```python
from build123d import *

# Parameters (mm, degrees)
SKETCH5_R             = 7
BOSS_EXTRUDE2_DEPTH   = 9.8
SKETCH6_R             = 10
BOSS_EXTRUDE3_DEPTH   = 7.2
M8_TAPPED_HOLE2_D     = 6.8
M8_TAPPED_HOLE2_DEPTH = 17
M8_TAPPED_HOLE2_TIP   = 2.042926105
BOSS_EXTRUDE5_DEPTH   = 8
SKETCH12_R            = 2.75
CUT_EXTRUDE6_DEPTH    = 9
M2_TAPPED_HOLE1_D     = 1.6
M2_TAPPED_HOLE1_DEPTH = 5.2
M2_TAPPED_HOLE1_TIP   = 0.480688495


with BuildPart() as part:
    # Sketch5 → Boss-Extrude2 (new body)
    with BuildSketch(Plane(origin=(0, 0, 0), x_dir=(1, 0, 0), z_dir=(0, 1, 0))):
        Circle(SKETCH5_R)
    extrude(amount=BOSS_EXTRUDE2_DEPTH)

    # Sketch6 → Boss-Extrude3 (add)
    with BuildSketch(Plane(origin=(0, 9.8, 0), x_dir=(1, 0, 0), z_dir=(0, 1, 0))):
        Circle(SKETCH6_R)
    extrude(amount=BOSS_EXTRUDE3_DEPTH)

    # M8 Tapped Hole2
    with Locations(Plane(origin=(0, 0, 0), x_dir=(-1, 0, 0), z_dir=(0, -1, 0))):
        with Locations((0, 0)):
            Hole(M8_TAPPED_HOLE2_D / 2, depth=M8_TAPPED_HOLE2_DEPTH)
            with Locations((0, 0, -(M8_TAPPED_HOLE2_DEPTH + M8_TAPPED_HOLE2_TIP / 2))):  # 118° drill point
                Cone(0, M8_TAPPED_HOLE2_D / 2, M8_TAPPED_HOLE2_TIP, mode=Mode.SUBTRACT)

    # Sketch11 → Boss-Extrude5 (add)
    with BuildSketch(Plane(origin=(0, 17, 0), x_dir=(1, 0, 0), z_dir=(0, 1, 0))):
        with BuildLine():
            Line((-5.5, 2.397915762), (-5.5, -2.397915762))
            ThreePointArc((-5.5, -2.397915762), (6, 0), (-5.5, 2.397915762))
        make_face()
    extrude(amount=BOSS_EXTRUDE5_DEPTH)

    # Sketch12 → Cut-Extrude6 (cut)
    with BuildSketch(Plane(origin=(0, 25, 0), x_dir=(1, 0, 0), z_dir=(0, 1, 0))):
        Circle(SKETCH12_R)
    extrude(amount=-CUT_EXTRUDE6_DEPTH, mode=Mode.SUBTRACT)

    # M2 Tapped Hole1
    with Locations(Plane.ZY.offset(5.5)):
        with Locations((0, 21.552134156)):
            Hole(M2_TAPPED_HOLE1_D / 2, depth=M2_TAPPED_HOLE1_DEPTH)
            with Locations((0, 0, -(M2_TAPPED_HOLE1_DEPTH + M2_TAPPED_HOLE1_TIP / 2))):  # 118° drill point
                Cone(0, M2_TAPPED_HOLE1_D / 2, M2_TAPPED_HOLE1_TIP, mode=Mode.SUBTRACT)


solid = part.part
```
Geometry check sheet. Reference: the model listing, model coordinates, mm. A direction names the side the tool comes from. Coordinates: 2 decimals unless noted, no trailing zeros. Order: outer loops, then holes, each group sorted by start corner. A loop starts at its lowest first (then second) coordinate and runs counter-clockwise, first axis right, second up. Notation, with made-up numbers: (14.5, 58) - (71.5, 58) arc R12 cw to (71.5, 80) - close; hole circle Ø4 at (50.25, 57.5). An arc over 180 degrees is marked (long way). Use one line per item in the form item = value.
1. Section check A-A (z = 0). Record the boundary of the cut face in (x, y), then the cut area to 3 significant figures.
Here are the results:
outline = (-10, 9.8) - (-7, 9.8) - (-7, 0) - (-3.4, 0) - (-3.4, 17) - (-2.75, 17) - (-2.75, 20.75) - (-5.5, 20.75) - (-5.5, 17) - (-10, 17) - close; (-5.5, 22.35) - (-2.75, 22.35) - (-2.75, 25) - (-5.5, 25) - close; (2.75, 17) - (3.4, 17) - (3.4, 0) - (7, 0) - (7, 9.8) - (10, 9.8) - (10, 17) - (6, 17) - (6, 25) - (2.75, 25) - close
area = 209 mm²
2. Draft check along X on faces 1 (the face through (-5.5, 21, -1)), 2 (the face through (0, 17, 7)), 3 (the face through (3, 17, 0)), 4 (the face through (2.54, 21.06, 1.05)). Enter one of: pulls with the +X half, pulls with the -X half, needs draft (parallel to the pull), parting line crosses it, or undercut.
Here are the results:
face_1 = pulls with the -X half
face_2 = needs draft
face_3 = undercut
face_4 = undercut
3. Gauge pin test, flat ends, axial feed: pin 1 (1.5 mm diameter, centred on x = -4, y = 14.5, fed in from -Z); pin 2 (6 mm diameter, centred on x = -4.5, y = 4, fed in from +Z); pin 3 (1 mm diameter, centred on y = 21.55, z = 0, fed in from -X). Record the tip position at first contact, or that the pin passes through.
Here are the results:
pin_1 = -9.46
pin_2 = 6.84
pin_3 = 2.7
4. Section check B-B (x = 0). Record the boundary of the cut face in (y, z).
Here are the results:
outline = (0, -7) - (9.8, -7) - (9.8, -10) - (17, -10) - (17, -6) - (25, -6) - (25, -2.75) - (17, -2.75) - (17, -3.4) - (0, -3.4) - close; (0, 3.4) - (17, 3.4) - (17, 2.75) - (25, 2.75) - (25, 6) - (17, 6) - (17, 10) - (9.8, 10) - (9.8, 7) - (0, 7) - close
5. Access from +Z, -Z, +X, -X, +Y, -Y to the whole of each face (thin tool, end or side, straight path). Record for faces 5 (the face through (-4.045, 22.345, 0.104)), 6 (the face through (-7, 9.8, 2)), 7 (the face through (3, 0, -2)), 8 (the face through (6, 21, 0)).
Here are the results:
face_5 = -X
face_6 = -Y
face_7 = +Z, -Z, +X, -X, -Y
face_8 = +Y
6. Section check C-C (y = 9). Record the boundary of the cut face in (x, z), then the cut area to 3 significant figures.
Here are the results:
outline = circle Ø14 at (0, 0); hole circle Ø6.8 at (0, 0)
area = 118 mm²
7. Scan lines: line 1 (X direction, y = 18.5, z = 0); line 2 (Z direction, x = 0, y = 16.5); line 3 (Z direction, x = 0, y = 22.25). Record each from-to range of solid material in increasing order.
Here are the results:
line_1 = -5.5 to -2.75, 2.75 to 6
line_2 = -10 to -3.4, 3.4 to 10
line_3 = -6 to -2.75, 2.75 to 6
8. Section check D-D (x = -6). Record the boundary of the cut face in (y, z).
Here are the results:
outline = (0, -3.61) - (9.8, -3.61) - (9.8, -8) - (17, -8) - (17, 8) - (9.8, 8) - (9.8, 3.61) - (0, 3.61) - close
